```python
from build123d import *

# Parameters (mm, degrees)
SKETCH1_W           = 250
SKETCH1_H           = 250
BOSS_EXTRUDE1_DEPTH = 50
BOSS_EXTRUDE2_DEPTH = 20
SKETCH3_R           = 5
CUT_EXTRUDE1_DEPTH  = 25
SKETCH5_W           = 242
SKETCH5_H           = 242
CUT_EXTRUDE2_DEPTH  = 46
FILLET1_R           = 10
FILLET2_R           = 10


with BuildPart() as part:
    # Sketch1 → Boss-Extrude1 (new body)
    with BuildSketch(Plane.XY):
        with Locations((125, 125)):
            Rectangle(SKETCH1_W, SKETCH1_H)
    extrude(amount=BOSS_EXTRUDE1_DEPTH)

    # Sketch2 → Boss-Extrude2 (add)
    with BuildSketch(Plane.XY):
        with BuildLine():
            Line((105, 0), (105, -15))
            ThreePointArc((105, -15), (105.585786438, -16.414213562), (107, -17))
            Line((107, -17), (143, -17))
            ThreePointArc((143, -17), (144.414213562, -16.414213562), (145, -15))
            Line((145, -15), (145, 0))
            Line((145, 0), (105, 0))
        make_face()
    boss_extrude2 = extrude(amount=BOSS_EXTRUDE2_DEPTH)

    # Mirror1: Boss-Extrude2 across plane
    add(boss_extrude2.mirror(Plane.ZX.offset(125)))

    # Sketch3 → Cut-Extrude1 (cut)
    with BuildSketch(Plane(origin=(0, 0, 0), x_dir=(-1, 0, 0), z_dir=(0, 0, -1))):
        with Locations((-125, -7.5)):
            Circle(SKETCH3_R)
        with Locations((-125, 257.5)):
            Circle(SKETCH3_R)
    extrude(amount=-CUT_EXTRUDE1_DEPTH, mode=Mode.SUBTRACT)

    # Sketch5 → Cut-Extrude2 (cut)
    with BuildSketch(Plane(origin=(0, 0, 0), x_dir=(-1, 0, 0), z_dir=(0, 0, -1))):
        with Locations((-125, 125)):
            Rectangle(SKETCH5_W, SKETCH5_H)
    extrude(amount=-CUT_EXTRUDE2_DEPTH, mode=Mode.SUBTRACT)

    # Fillet1
    fillet1_edges = [part.edges().sort_by_distance(p)[0] for p in [
        (0, 250, 25),
        (250, 250, 25),
        (250, 0, 25),
        (0, 0, 25),
    ]]
    fillet(fillet1_edges, radius=FILLET1_R)

    # Fillet2
    fillet2_edges = [part.edges().sort_by_distance(p)[0] for p in [
        (246, 246, 23),
        (4, 246, 23),
        (4, 4, 23),
        (246, 4, 23),
    ]]
    fillet(fillet2_edges, radius=FILLET2_R)


solid = part.part
```
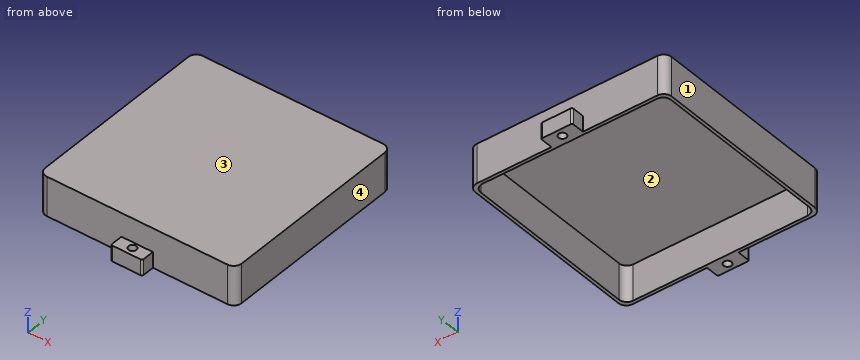
Could you check a few things on this model? Use its own coordinates, in mm. Face numbers are marked on the shaded views. Round coordinates to 2 decimals unless told otherwise and drop trailing zeros. Order: outer loops, then holes, each group sorted by start corner. A loop starts at its lowest first (then second) coordinate and runs counter-clockwise, first axis right, second up. Notation, with made-up numbers: (62, 78.25) -> (77, 78.25) arc R19 cw to (77, 99.25) -> close; hole circle Ø3 at (41, 51.25). An arc over 180 degrees is marked (long way). One line per question, with ' | ' between items.
Q1. I'm going to push flat-ended pins straight in: pin 1 (1.5 mm diameter, centred on x = 211, z = 17, fed in from +Y); pin 2 (13 mm diameter, centred on x = 125, y = -7.5, fed in from +Z); pin 3 (4.5 mm diameter, centred on y = -4.5, z = 9.5, fed in from -X). Where does each tip first touch, or does it pass through?
Computed values:
pin 1: y = 250 | pin 2: z = 20 | pin 3: x = 105
Q2. If we section it at C-C on z = 28: Write out the boundary of the cut face in (x, y).
Computed values:
outline: (0, 10) arc R10 ccw to (10, 0) -> (240, 0) arc R10 ccw to (250, 10) -> (250, 240) arc R10 ccw to (240, 250) -> (10, 250) arc R10 ccw to (0, 240) -> close; hole (4, 14) arc R10 ccw to (14, 4) -> (236, 4) arc R10 ccw to (246, 14) -> (246, 236) arc R10 ccw to (236, 246) -> (14, 246) arc R10 ccw to (4, 236) -> close
Q3. We'd pull the mould along X, two halves only. Please class the marked faces 1, 2, 3 and 4: released by +X, released by -X, zero draft, split by the parting line, or undercut.
Computed values:
face 1: released by -X | face 2: undercut | face 3: zero draft | face 4: released by +X
Q4. If we section it at A-A on y = 257.5: Write out the boundary of the cut face in (x, z).
Computed values:
outline: (105, 0) -> (120, 0) -> (120, 20) -> (105, 20) -> close; (130, 0) -> (145, 0) -> (145, 20) -> (130, 20) -> close
Q5. If we section it at B-B on x = 125: Write out the boundary of the cut face in (y, z).
Computed values:
outline: (-17, 0) -> (-12.5, 0) -> (-12.5, 20) -> (-17, 20) -> close; (-2.5, 0) -> (4, 0) -> (4, 46) -> (246, 46) -> (246, 0) -> (252.5, 0) -> (252.5, 20) -> (250, 20) -> (250, 50) -> (0, 50) -> (0, 20) -> (-2.5, 20) -> close; (262.5, 0) -> (267, 0) -> (267, 20) -> (262.5, 20) -> close
Q6. If we section it at D-D on y = 186.5: Write out the boundary of the cut face in (x, z), plus the area to 3 significant figures.
Computed values:
outline: (0, 0) -> (4, 0) -> (4, 46) -> (246, 46) -> (246, 0) -> (250, 0) -> (250, 50) -> (0, 50) -> close | area: 1,370 mm²
Q7. If I drill on line 1 (Y direction, x = 125, z = 15); line 2 (X direction, y = 52.5, z = 45), over which ranges is the centre line in solid material (lowest first)? Write a range as from..to.
Computed values:
line 1: -17..-12.5, -2.5..4, 246..252.5, 262.5..267 | line 2: 0..4, 246..250
